Could you check a few things on this model? Use its own coordinates, in mm. A direction names the side the tool comes from. Give positions to 0.01 mm unless a question says otherwise; leave off trailing zeros. Loops run counter-clockwise (first coordinate to the right, second up) from the corner with the lowest first, then second, coordinate; pieces in that order, holes last. Notation, with made-up numbers: M -6.75,-6 L 12.25,-6 A23 cw 12.25,28 Z; hole C 44,38.5 d9. An arc over 180 degrees is marked long. Answer in a Markdown table with one row per item. Add a question column.
1. I need wall thicknesses on line 1 along Y through (x, z) = (503, 5.75); line 2 along Y through (x, z) = (627, 1.25); line 3 along Y through (x, z) = (993, 4.25). Which ranges of each line are inside material? Lowest first, please. Write a range as from..to.
2. If we section it at A-A on x = 432.5: List the corners of the cut face in (y, z) for me, then the cut area to 3 significant figures.
3. Thinking about a two-plate mould opening in X: for faces 1 (the flat face through (1005, 206, 10)), 2 (the cylindrical face through (1664.742, 429.964, 4.93)), which applies, released by +X, released by -X, zero draft, split by the parting line, or undercut?
4. If we section it at B-B on x = 1002: List the corners of the cut face in (y, z) for me, then the cut area to 3 significant figures.
5. Which directions (+Z, -Z, +X, -X, +Y, -Y) give clear straight access to the entire face, cutting with the end or side of a thin tool? Please do faces 3 (the flat face through (1005, 206, 0)), 4 (the cylindrical face through (1663.964, 332.258, 4.93)).
6. If we section it at C-C on z = 6: Count the separate pieces of the cut face and the enclosed holes in it, then the cut area to 3 significant figures.
```python
from build123d import *

# Parameters (mm, degrees)
SKETCH_W   = 2038
SKETCH_H   = 520
SKETCH_W_2 = 216
SKETCH_H_2 = 24
PAD_DEPTH  = 10


with BuildPart() as part:
    # Sketch → Pad (new body)
    with BuildSketch(Plane.XY):
        with Locations((1019, 260)):
            Rectangle(SKETCH_W, SKETCH_H)
        with BuildLine():
            Line((359, 395), (359, 368))
            ThreePointArc((359, 368), (373.644661, 332.644661), (409, 318))
            Line((409, 318), (625, 318))
            ThreePointArc((625, 318), (660.355339, 332.644661), (675, 368))
            Line((675, 368), (675, 395))
            ThreePointArc((675, 395), (660.355339, 430.355339), (625, 445))
            Line((625, 445), (409, 445))
            ThreePointArc((409, 445), (373.644661, 430.355339), (359, 395))
        make_face(mode=Mode.SUBTRACT)
        with BuildLine():
            Line((1363, 395), (1363, 368))
            ThreePointArc((1363, 368), (1377.644661, 332.644661), (1413, 318))
            Line((1413, 318), (1629, 318))
            ThreePointArc((1629, 318), (1664.355339, 332.644661), (1679, 368))
            Line((1679, 368), (1679, 395))
            ThreePointArc((1679, 395), (1664.355339, 430.355339), (1629, 445))
            Line((1629, 445), (1413, 445))
            ThreePointArc((1413, 445), (1377.644661, 430.355339), (1363, 395))
        make_face(mode=Mode.SUBTRACT)
        with BuildLine():
            Line((359, 156.0146), (359, 129.0146))
            ThreePointArc((359, 129.0146), (373.644661, 93.659261), (409, 79.0146))
            Line((409, 79.0146), (625, 79.0146))
            ThreePointArc((625, 79.0146), (660.355339, 93.659261), (675, 129.0146))
            Line((675, 129.0146), (675, 156.0146))
            ThreePointArc((675, 156.0146), (660.355339, 191.369939), (625, 206.0146))
            Line((625, 206.0146), (409, 206.0146))
            ThreePointArc((409, 206.0146), (373.644661, 191.369939), (359, 156.0146))
        make_face(mode=Mode.SUBTRACT)
        with BuildLine():
            Line((1363, 156.0146), (1363, 129.0146))
            ThreePointArc((1363, 129.0146), (1377.644661, 93.659261), (1413, 79.0146))
            Line((1413, 79.0146), (1629, 79.0146))
            ThreePointArc((1629, 79.0146), (1664.355339, 93.659261), (1679, 129.0146))
            Line((1679, 129.0146), (1679, 156.0146))
            ThreePointArc((1679, 156.0146), (1664.355339, 191.369939), (1629, 206.0146))
            Line((1629, 206.0146), (1413, 206.0146))
            ThreePointArc((1413, 206.0146), (1377.644661, 191.369939), (1363, 156.0146))
        make_face(mode=Mode.SUBTRACT)
        with Locations((1019, 260)):
            Rectangle(SKETCH_W_2, SKETCH_H_2, mode=Mode.SUBTRACT)
    extrude(amount=PAD_DEPTH)


solid = part.part
```
Results:
| question | item | result |
|---|---|---|
| 1 | line 1 | 0..79.01, 206.01..318, 445..520 |
| 1 | line 2 | 0..79.05, 205.97..318.04, 444.96..520 |
| 1 | line 3 | 0..248, 272..520 |
| 2 | outline | M 0,0 L 79.01,0 L 79.01,10 L 0,10 Z; M 206.01,0 L 318,0 L 318,10 L 206.01,10 Z; M 445,0 L 520,0 L 520,10 L 445,10 Z |
| 2 | area | 2,660 mm2 |
| 3 | face 1 | zero draft |
| 3 | face 2 | undercut |
| 4 | outline | M 0,0 L 248,0 L 248,10 L 0,10 Z; M 272,0 L 520,0 L 520,10 L 272,10 Z |
| 4 | area | 4,960 mm2 |
| 5 | face 3 | -Z, +X, -X, +Y, -Y |
| 5 | face 4 | +Z, -Z |
| 6 | separate pieces | 1 |
| 6 | enclosed holes | 5 |
| 6 | area | 903,000 mm2 |
